from build123d import *

# Parameters (mm, degrees)
F1_DEPTH = 3


with BuildPart() as f1:
    # F0 (on Front) → F1 (new body)
    with BuildSketch(Plane.XZ):
        with BuildLine():
            Line((-171.156163, -50), (-171.156163, 0))
            Line((-171.156163, 0), (-171.156163, 30))
            ThreePointArc((-171.156163, 30), (-174.085096, 37.071068), (-181.156163, 40))
            Line((-181.156163, 40), (-216.156163, 40))
            Line((-216.156163, 40), (-216.156163, -90))
            Line((-216.156163, -90), (-181.156163, -90))
            ThreePointArc((-181.156163, -90), (-174.085096, -87.071068), (-171.156163, -80))
            Line((-171.156163, -80), (-171.156163, -50))
        make_face()
        with BuildLine():
            Line((-192.156163, -58), (-192.156163, -70))
            ThreePointArc((-192.156163, -70), (-196.156163, -74), (-200.156163, -70))
            Line((-200.156163, -70), (-200.156163, -58))
            ThreePointArc((-200.156163, -58), (-196.156163, -54), (-192.156163, -58))
        make_face(mode=Mode.SUBTRACT)
        with BuildLine():
            Line((-200.156163, 8), (-200.156163, 20))
            ThreePointArc((-200.156163, 20), (-196.156163, 24), (-192.156163, 20))
            Line((-192.156163, 20), (-192.156163, 8))
            ThreePointArc((-192.156163, 8), (-196.156163, 4), (-200.156163, 8))
        make_face(mode=Mode.SUBTRACT)
        with BuildLine():
            Line((-101.156163, 0), (-171.156163, 0))
            Line((-171.156163, 0), (-171.156163, -50))
            Line((-171.156163, -50), (419.01048, -40.163889))
            ThreePointArc((419.01048, -40.163889), (425.973578, -37.177181), (428.843837, -30.165278))
            Line((428.843837, -30.165278), (428.843837, 0))
            Line((428.843837, 0), (423.843837, 0))
            Line((423.843837, 0), (423.843837, -25))
            Line((423.843837, -25), (398.843837, -25))
            Line((398.843837, -25), (398.843837, 0))
            Line((398.843837, 0), (298.843837, 0))
            Line((298.843837, 0), (298.843837, -25))
            Line((298.843837, -25), (273.843837, -25))
            Line((273.843837, -25), (273.843837, 0))
            Line((273.843837, 0), (173.843837, 0))
            Line((173.843837, 0), (173.843837, -25))
            Line((173.843837, -25), (163.126186, -25))
            Line((163.126186, -25), (148.843837, -25))
            Line((148.843837, -25), (148.843837, 0))
            Line((148.843837, 0), (48.843837, 0))
            Line((48.843837, 0), (48.843837, -25))
            Line((48.843837, -25), (23.843837, -25))
            Line((23.843837, -25), (23.843837, 0))
            Line((23.843837, 0), (-76.156163, 0))
            Line((-76.156163, 0), (-76.156163, -25))
            Line((-76.156163, -25), (-101.156163, -25))
            Line((-101.156163, -25), (-101.156163, 0))
        make_face()
    extrude(amount=F1_DEPTH)


solid = f1.part
Build history of the part. All positions in model axes, mm. Coordinates: 2 decimals unless noted, no trailing zeros. Write each loop counter-clockwise with the first axis right and the second up, starting at its lowest first coordinate (ties: lowest second). Pieces come first, ordered by that corner, then holes. Notation, with made-up numbers: (28.25, 70.5) -> (58.25, 70.5) arc R12 ccw to (58.25, 87.5) -> close; hole circle Ø5 at (34, 14). An arc over 180 degrees is marked (long way). Use CSV: the item, a comma, the result in double quotes. Start each with the question number.
Q1. Cut at C-C, the plane x = 346.5. List the corners of the cut face in (y, z).
Q2. Cut at A-A, the plane z = -9.5. List the corners of the cut face in (x, y).
Q3. Flat gauge pins, fed straight in: pin 1 Ø0.9 at (y, z) = (-1.5, 22) entering from +X; pin 2 Ø1.5 at (x, y) = (236, -2) entering from +Z. Where does each tip first touch, or does it go through?
Q4. Cut at B-B, the plane y = -1. State how many separate pieces and enclosed holes the cut face has, then the cut area to 3 significant figures.
Q5. Cut at D-D, the plane x = 110. List the corners of the cut face in (y, z), then the cut area to 3 significant figures.
Q6. Drill centre lines: probe 1 along X at (y, z) = (-1.75, -18); probe 2 along X at (y, z) = (-2.65, -57); probe 3 along X at (y, z) = (-2.4, 19.5). Where is each one in solid material? Low to high.
Checked values:
1,outline,"(-3, -41.37) -> (0, -41.37) -> (0, 0) -> (-3, 0) -> close"
2,outline,"(-216.16, -3) -> (-101.16, -3) -> (-101.16, 0) -> (-216.16, 0) -> close; (-76.16, -3) -> (23.84, -3) -> (23.84, 0) -> (-76.16, 0) -> close; (48.84, -3) -> (148.84, -3) -> (148.84, 0) -> (48.84, 0) -> close; (173.84, -3) -> (273.84, -3) -> (273.84, 0) -> (173.84, 0) -> close; (298.84, -3) -> (398.84, -3) -> (398.84, 0) -> (298.84, 0) -> close; (423.84, -3) -> (428.84, -3) -> (428.84, 0) -> (423.84, 0) -> close"
3,pin 1,"stops at x = -171.16"
3,pin 2,"stops at z = 0"
4,separate pieces,"1"
4,enclosed holes,"2"
4,area,"29,400 mm²"
5,outline,"(-3, -45.31) -> (0, -45.31) -> (0, 0) -> (-3, 0) -> close"
5,area,"136 mm²"
6,probe 1,"x = -216.16 to -101.16, -76.16 to 23.84, 48.84 to 148.84, 173.84 to 273.84, 298.84 to 398.84, 423.84 to 428.84"
6,probe 2,"x = -216.16 to -200.03, -192.28 to -171.16"
6,probe 3,"x = -216.16 to -200.16, -192.16 to -171.16"
